Source: CAD feature listing. Evaluate the final solid. Frame: model axes, mm. A direction names the side the tool comes from. Give positions to 0.01 mm unless a question says otherwise; leave off trailing zeros. Loops run counter-clockwise (first coordinate to the right, second up) from the corner with the lowest first, then second, coordinate; pieces in that order, holes last. Notation, with made-up numbers: (2.25, 21.25) -> (59.25, 21.25) arc R19 cw to (59.25, 52.25) -> close; hole circle Ø4 at (54, 64). An arc over 180 degrees is marked (long way). Put each result on its own line as item: value.
```python
from build123d import *

# Parameters (mm, degrees)
EXTRUDE003_DEPTH                  = 10
FILLET021_R                       = 1
EXTRUDE004_DEPTH                  = 5
PART_MIRRORING006_PLACEMENT_ANGLE = 180


with BuildPart() as fillet021:
    # Sketch005 → Extrude003 (new body)
    with BuildSketch(Plane.XY):
        Polygon((57.709053, -19.346786), (57.709053, -22.346786), (65.709053, -22.346786), (65.709053, -10.346786), (62.709053, -10.346786), (62.709053, -19.346786), align=None)
    extrude(amount=EXTRUDE003_DEPTH)


with BuildPart() as fillet021_1:
    # Extrude003 placement: moved
    add(fillet021.part.moved(Location((0, 0, -14))))

    # Fillet021
    fillet021_edges = [fillet021_1.edges().sort_by_distance(p)[0] for p in [
        (57.709053, -19.346786, -9),
        (57.709053, -22.346786, -9),
        (65.709053, -22.346786, -9),
        (61.709053, -22.346786, -4),
        (65.709053, -10.346786, -9),
        (65.709053, -16.346786, -4),
        (62.709053, -10.346786, -9),
        (64.209053, -10.346786, -4),
        (62.709053, -19.346786, -9),
        (62.709053, -14.846786, -4),
        (60.209053, -19.346786, -4),
    ]]
    fillet(fillet021_edges, radius=FILLET021_R)


with BuildPart() as fillet021_2:
    # Fillet021 placement: moved
    add(fillet021_1.part.moved(Location((0, 0, 0.4))))


with BuildPart() as extrude004:
    # Sketch006 → Extrude004 (new body)
    with BuildSketch(Plane.XZ):
        with BuildLine():
            ThreePointArc((14.771842, 0.154152), (17.827348, 3.62591), (14.461083, 6.797264))
            Line((14.461083, 6.797264), (12.252875, 6.797264))
            Line((12.252875, -5.267611), (12.252875, 6.797264))
            Line((5.422805, -5.82309), (12.252875, -5.267611))
            ThreePointArc((5.422805, -5.82309), (2.802341, -9.576998), (6.556249, -12.197462))
            Line((6.556249, -12.197462), (14.771842, -12.197462))
            Line((14.771842, -12.197462), (14.771842, 0.154152))
        make_face()
    extrude(amount=EXTRUDE004_DEPTH)


with BuildPart() as extrude004_1:
    # Extrude004 placement: moved
    add(extrude004.part.moved(Location((0, -8, 0))))


with BuildPart() as c4holds003:
    # Part__Mirroring006: instance of Extrude004
    add(extrude004_1.part.mirror(Plane(origin=(0, 0, 0), x_dir=(0, 1, 0), z_dir=(0, 0, 1))))


with BuildPart() as c4holds003_1:
    # Part__Mirroring006 placement: moved
    add(c4holds003.part.moved(Location((78, 0, 0))).rotate(Axis((78, 0, 0), (0, 1, 0)), PART_MIRRORING006_PLACEMENT_ANGLE))

    # Fusion041: union Fillet021
    add(fillet021_2.part)


solid = c4holds003_1.part
```
(1) Draft query along Z for faces 5 (the flat face through (63, -18, -13.6)), 6 (the flat face through (68, -13, -6)), 7 (the cylindrical face through (75.21, -10.46, -9.51)), 8 (the flat face through (63.228, -10, -5)). Return one class per face: released by +Z, released by -Z, zero draft, split by the parting line, or undercut.
Calculated:
face 5: released by -Z
face 6: zero draft
face 7: split by the parting line
face 8: undercut
(2) Section A-A on y = -12.75. Return loops of the section in (x, z).
Calculated:
outline: (62.71, -13.6) -> (65.71, -13.6) -> (65.71, -12.2) -> (71.44, -12.2) arc R3.24 ccw to (72.58, -5.82) -> (65.75, -5.27) -> (65.75, 6.8) -> (63.54, 6.8) arc R3.33 ccw to (63.23, 0.15) -> (63.23, -3.72) arc R1 ccw to (62.71, -4.6) -> close
(3) First-contact query: P1, Ø1.5, axis at y = -10.5, z = -5, coming from the -X side; P2, Ø5.5, axis at y = -10, z = 4, coming from the +X side; P3, Ø2, axis at x = 72.5, z = -8.5, coming from the -Y side. Flat tips, straight axial feed; report the tip coordinate or a pass-through.
Calculated:
P1: stops at x = 62.71
P2: stops at x = 65.75
P3: stops at y = -13
(4) Line query: probe 1 along X at (y, z) = (-21.25, -8.75); probe 2 along Y at (x, z) = (61.5, -6.25); probe 3 along X at (y, z) = (-13.5, -8.25). Output: solid intervals per line, ascending. Write a range as from..to.
Calculated:
probe 1: x = 57.71..65.71
probe 2: y = -22.35..-19.35
probe 3: x = 62.71..65.71
(5) Reachability of faces 1 (the flat face through (68, -10, -12.197)), 2 (the flat face through (60, -19.347, -9)), 3 (the cylindrical face through (65.424, -17.115, -3.901)), 4 (the flat face through (65.747, -10, 1)) from +Z, -Z, +X, -X, +Y, -Y: full face, straight path, thin tool, end or side. Return the list, or none.
Calculated:
face 1: -Z, +Y
face 2: +Z, -Z, -X, +Y
face 3: +Z, +X, -Y
face 4: +Z, +X, +Y, -Y
(6) Section D-D on y = -9.25. Return loops of the section in (x, z), then the cut area to 3 significant figures.
Calculated:
outline: (63.23, -12.2) -> (71.44, -12.2) arc R3.24 ccw to (72.58, -5.82) -> (65.75, -5.27) -> (65.75, 6.8) -> (63.54, 6.8) arc R3.33 ccw to (63.23, 0.15) -> close
area: 122 mm²
(7) Section C-C on z = -2.5. Return loops of the section in (x, y), then the cut area to 3 significant figures.
Calculated:
outline: (63.23, -13) -> (65.75, -13) -> (65.75, -8) -> (63.23, -8) -> close
area: 12.6 mm²
(8) Section B-B on x = 60.75. Return loops of the section in (y, z).
Calculated:
outline: (-22.35, -13.6) -> (-19.35, -13.6) -> (-19.35, -4.6) arc R1 ccw to (-20.35, -3.6) -> (-21.35, -3.6) arc R1 ccw to (-22.35, -4.6) -> close; (-13, 1.59) -> (-8, 1.59) -> (-8, 5.35) -> (-13, 5.35) -> close
